Could you check a few things on this drawing? It's one solid part, dimensions in mm from its lowest x, y, z. A direction names the side the tool comes from. Give positions to 0.01 mm unless a question says otherwise; leave off trailing zeros. Loops run counter-clockwise (first coordinate to the right, second up) from the corner with the lowest first, then second, coordinate; pieces in that order, holes last. Notation, with made-up numbers: (42.25, 80) - (85.25, 80) arc R10 cw to (85.25, 93) - close; hole circle Ø2 at (24, -37). An arc over 180 degrees is marked (long way). Write item = value, one per line.
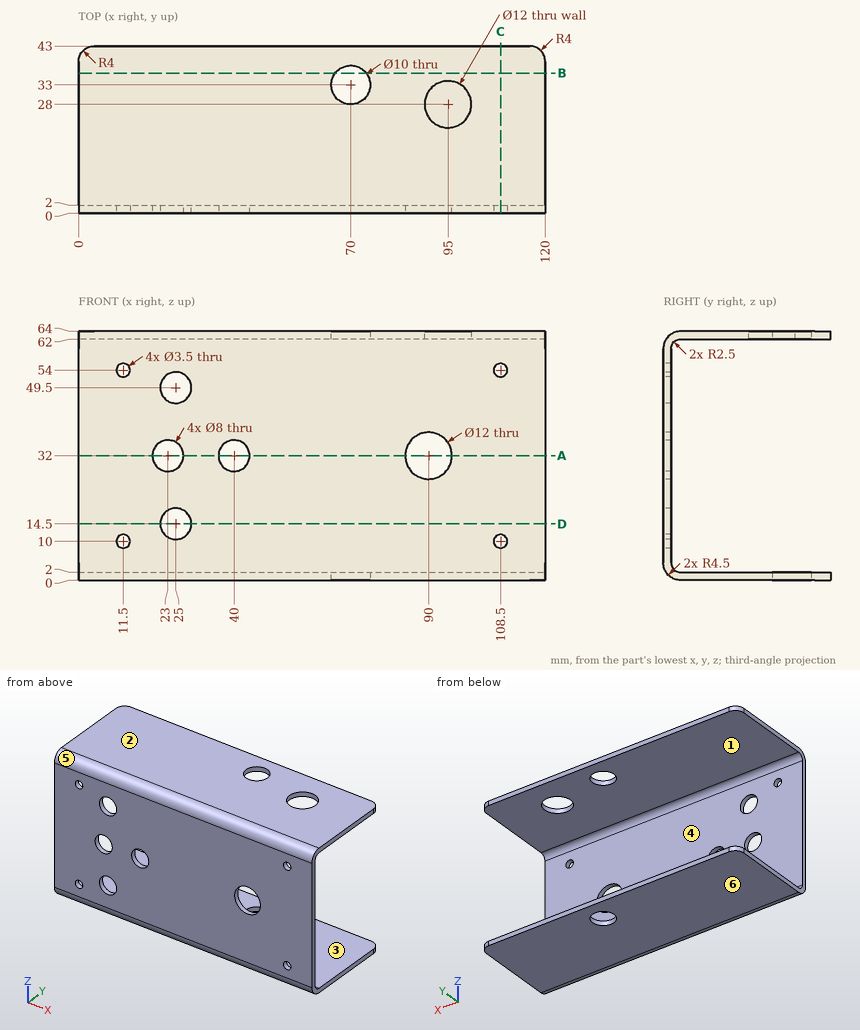
Q1. For pin 1 (8 mm diameter, centred on x = 70, y = 33, fed in from +Z); pin 2 (6 mm diameter, centred on x = 100.5, z = 12, fed in from +Y), each with a flat end and sliding along its axis, tell me the tip position at first contact or that it passes through.
Output:
pin_1 = through
pin_2 = 2
Q2. Imagine slicing it at C-C, the plane x = 108.5. Write out the boundary of the cut face in (y, z).
Output:
outline = (0, 4.5) arc R4.5 ccw to (4.5, 0) - (43, 0) - (43, 2) - (4.5, 2) arc R2.5 cw to (2, 4.5) - (2, 8.25) - (0, 8.25) - close; (0, 11.75) - (2, 11.75) - (2, 52.25) - (0, 52.25) - close; (0, 55.75) - (2, 55.75) - (2, 59.5) arc R2.5 cw to (4.5, 62) - (43, 62) - (43, 64) - (4.5, 64) arc R4.5 ccw to (0, 59.5) - close
Q3. Imagine slicing it at D-D, the plane z = 14.5. Write out the boundary of the cut face in (x, y).
Output:
outline = (0, 0) - (21, 0) - (21, 2) - (0, 2) - close; (29, 0) - (120, 0) - (120, 2) - (29, 2) - close
Q4. I need wall thicknesses on L1, parallel to X at y = 1, z = 54; L2, parallel to Z at x = 26.5, y = 31; L3, parallel to Z at x = 108.5, y = 0.95. Which ranges of each line are inside material? Lowest first, please.
Output:
L1 = 0 to 9.75, 13.25 to 106.75, 110.25 to 120
L2 = 0 to 2, 62 to 64
L3 = 1.73 to 8.25, 11.75 to 52.25, 55.75 to 62.27
Q5. Which directions (+Z, -Z, +X, -X, +Y, -Y) give clear straight access to the entire face, cutting with the end or side of a thin tool? Please do the marked faces 1 and 2.
Output:
face_1 = +X, -X, +Y
face_2 = +Z, +X, -X, +Y, -Y
Q6. Imagine slicing it at B-B, the plane y = 36. Write out the boundary of the cut face in (x, z), then the cut area to 3 significant figures.
Output:
outline = (0, 0) - (66, 0) - (66, 2) - (0, 2) - close; (0, 62) - (66, 62) - (66, 64) - (0, 64) - close; (74, 0) - (120, 0) - (120, 2) - (74, 2) - close; (74, 62) - (120, 62) - (120, 64) - (74, 64) - close
area = 448 mm2
Q7. Imagine slicing it at A-A, the plane z = 32. Write out the boundary of the cut face in (x, y).
Output:
outline = (0, 0) - (19, 0) - (19, 2) - (0, 2) - close; (27, 0) - (36, 0) - (36, 2) - (27, 2) - close; (44, 0) - (84, 0) - (84, 2) - (44, 2) - close; (96, 0) - (120, 0) - (120, 2) - (96, 2) - close
Q8. We'd pull the mould along Z, two halves only. Please class the marked faces 3, 4, 5 and 6: released by +Z, released by -Z, zero draft, split by the parting line, or undercut.
Output:
face_3 = undercut
face_4 = undercut
face_5 = released by +Z
face_6 = released by -Z
